Can you work these out from the model? Positions are in its coordinate system, mm. Face numbers are marked on the shaded views. A direction names the side the tool comes from. Coordinates: 2 decimals unless noted, no trailing zeros. Loops run counter-clockwise (first coordinate to the right, second up) from the corner with the lowest first, then second, coordinate; pieces in that order, holes last. Notation, with made-up numbers: (29, 67) -> (46, 67) arc R19 ccw to (46, 98) -> close; hole circle Ø1 at (68.5, 28). An arc over 180 degrees is marked (long way). Put each result on its own line as item: value. Start each with the question number.
Item 1: If we section it at D-D on y = 67.5: Please give me the cut outline in (x, z).
Item 2: If we section it at B-B on y = -122: Please give me the cut outline in (x, z), plus the area to 3 significant figures.
Item 3: For the marked faces 5 and 6, which set-ups out of +Z, -Z, +X, -X, +Y, -Y let a thin tool reach every point of the face, with its end or its side?
Item 4: If we section it at A-A on z = 52.5: Please give me the cut outline in (x, y).
Item 5: Please list where these lines run through material, in increasing order: L1, parallel to Y at x = 179, z = 259.5; L2, parallel to X at y = 195.5, z = 168; L3, parallel to Z at x = -61.5, y = -13.5. Write a range as from..to.
Item 6: If we section it at C-C on x = -174: Please give me the cut outline in (y, z).
Item 7: We'd pull the mould along Y, two halves only. Please class the marked faces 1, 2, 3 and 4: pulls with the +Y half, pulls with the -Y half, needs draft (parallel to the pull), parting line crosses it, or undercut.
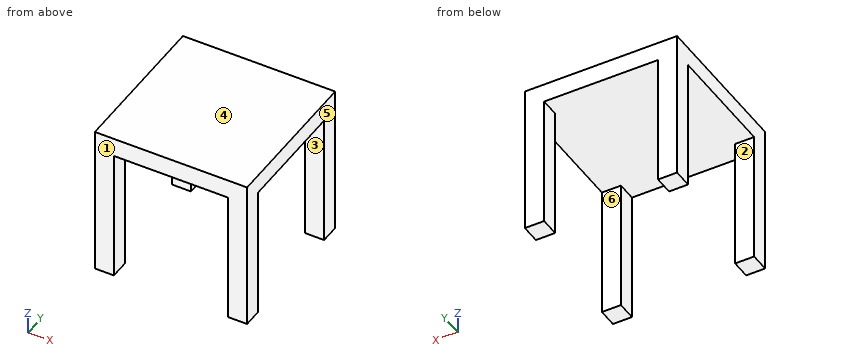
```python
from build123d import *

# Parameters (mm, degrees)
F0_W      = 400
F0_H      = 400
F1_DEPTH  = 350
F2_W      = 400
F2_H      = 50
F3_DEPTH  = 300
F5_DEPTH  = 50
F6_DEPTH  = 250
F7_DEPTH  = 250
F8_W      = 400
F8_H      = 96.5097817794
F9_DEPTH  = 300
F10_DEPTH = 50
F11_DEPTH = 350
F12_DEPTH = 345.44


with BuildPart() as f1:
    # F0 (on Top) → F1 (new body)
    with BuildSketch(Plane.XY):
        with Locations((-2.5529135019, 43.6986592397)):
            Rectangle(F0_W, F0_H)
    extrude(amount=F1_DEPTH)

    # F2 (on face) → F3 (join)
    with BuildSketch(Plane.XY.offset(350)):
        with Locations((-2.5529135019, 218.6986592397)):
            Rectangle(F2_W, F2_H)
    extrude(amount=F3_DEPTH)

    # F5 (add): a face of the model
    f5_faces = [f1.faces().sort_by_distance(p)[0] for p in [
        (-2.5529135019, 18.6986592397, 350),
    ]]
    extrude(f5_faces, amount=F5_DEPTH)

    # F6 (add): a face of the model
    f6_faces = [f1.faces().sort_by_distance(p)[0] for p in [
        (-2.5529135019, 218.6986592397, 650),
    ]]
    extrude(f6_faces, amount=-F6_DEPTH)

    # F7 (cut): a face of the model
    f7_faces = [f1.faces().sort_by_distance(p)[0] for p in [
        (-2.5529135019, 218.6986592397, 650),
    ]]
    extrude(f7_faces, amount=-F7_DEPTH, mode=Mode.SUBTRACT)

    # F8 (on face) → F9 (join)
    with BuildSketch(Plane.XY.offset(400)):
        with Locations((-2.5529135019, 291.9535501294)):
            Rectangle(F8_W, F8_H)
    extrude(amount=F9_DEPTH)

    # F10 (add): a face of the model
    f10_faces = [f1.faces().sort_by_distance(p)[0] for p in [
        (-2.5529135019, 243.6986592397, 550),
    ]]
    extrude(f10_faces, amount=-F10_DEPTH)

    # F4 (on face) → F11 (cut)
    with BuildSketch(Plane(origin=(0, 0, 0), x_dir=(1, 0, 0), z_dir=(0, 0, -1))):
        Polygon((147.4470864981, 156.3013407603), (-152.5529135019, 156.3013407603), (-152.5529135019, 106.3013407603), (-202.5529135019, 106.3013407603), (-202.5529135019, -193.6986592397), (-152.5529135019, -193.6986592397), (-152.5529135019, -243.6986592397), (146.7532366514, -243.6986592397), (146.7532366514, -193.6986592397), (197.4470864981, -193.6986592397), (197.4470864981, 106.3013407603), (147.4470864981, 106.3013407603), align=None)
    extrude(amount=-F11_DEPTH, mode=Mode.SUBTRACT)

    # F12 (cut): a face of the model
    f12_faces = [f1.faces().sort_by_distance(p)[0] for p in [
        (-2.5529135019, 291.9535501294, 700),
    ]]
    extrude(f12_faces, amount=-F12_DEPTH, mode=Mode.SUBTRACT)


solid = f1.part
```
Solutions:
1. outline: (-202.55, 350) -> (197.45, 350) -> (197.45, 400) -> (-202.55, 400) -> close
2. outline: (-202.55, 0) -> (-152.55, 0) -> (-152.55, 350) -> (147.45, 350) -> (147.45, 0) -> (197.45, 0) -> (197.45, 400) -> (-202.55, 400) -> close
2. area: 55,000 mm^2
3. face 5: +Z, -Z, +X, +Y, -Y
3. face 6: -Z, +X, -X
4. outline: (-202.55, -156.3) -> (-152.55, -156.3) -> (-152.55, -106.3) -> (-202.55, -106.3) -> close; (-202.55, 193.7) -> (-152.55, 193.7) -> (-152.55, 243.7) -> (-202.55, 243.7) -> close; (146.75, 193.7) -> (197.45, 193.7) -> (197.45, 243.7) -> (146.75, 243.7) -> close; (147.45, -156.3) -> (197.45, -156.3) -> (197.45, -106.3) -> (147.45, -106.3) -> close
5. L1: -156.3..-106.3, 193.7..243.7
5. L2: -202.55..-152.55, 146.75..197.45
5. L3: 350..400
6. outline: (-156.3, 0) -> (-106.3, 0) -> (-106.3, 350) -> (193.7, 350) -> (193.7, 0) -> (243.7, 0) -> (243.7, 400) -> (-156.3, 400) -> close
7. face 1: pulls with the -Y half
7. face 2: undercut
7. face 3: undercut
7. face 4: needs draft
